from build123d import *

# Parameters (mm, degrees)
F1_DEPTH = 70
F3_DEPTH = 5


with BuildPart() as f1:
    # F0 (on Front) → F1 (new body)
    with BuildSketch(Plane.XZ):
        Polygon((0, 3), (0, 0), (25, 0), (25, -20.415811), (25, -22.415811), (30, -22), (30, 3), align=None)
        Polygon((25, -22.415811), (25, -20.415811), (0, -22.494866), (0, -24.494866), align=None)
    extrude(amount=F1_DEPTH)

    # F2 (on face) → F3 (cut)
    with BuildSketch(Plane.XY.offset(3)):
        with BuildLine():
            ThreePointArc((19, -14.5), (17.828427, -11.671573), (15, -10.5))
            Line((15, -10.5), (15, -14.5))
            Line((15, -14.5), (15, -18.5))
            ThreePointArc((15, -18.5), (17.828427, -17.328427), (19, -14.5))
        make_face()
        with BuildLine():
            ThreePointArc((19, -55.5), (17.828427, -52.671573), (15, -51.5))
            ThreePointArc((15, -51.5), (12.171573, -58.328427), (19, -55.5))
        make_face()
        with BuildLine():
            Line((15, -14.5), (15, -10.5))
            ThreePointArc((15, -10.5), (11, -14.5), (15, -18.5))
            Line((15, -18.5), (15, -14.5))
        make_face()
    extrude(amount=-F3_DEPTH, mode=Mode.SUBTRACT)


solid = f1.part
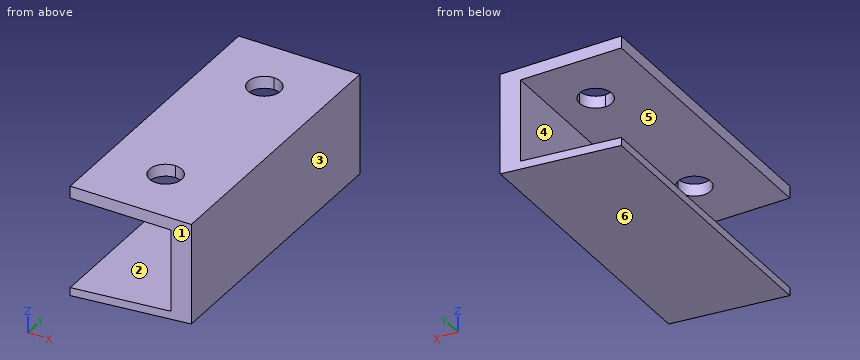
CAD build for the part. Positions are in the model's coordinates, mm. Face numbers are marked on the shaded views. A direction names the side the tool comes from. Give positions to 0.01 mm unless a question says otherwise; leave off trailing zeros. Write each loop counter-clockwise with the first axis right and the second up, starting at its lowest first coordinate (ties: lowest second). Pieces come first, ordered by that corner, then holes. Notation, with made-up numbers: (-19, -26.75) - (0, -26.75) arc R10 ccw to (0, -14.75) - close; hole circle Ø4 at (-18, -25). An arc over 180 degrees is marked (long way). Put each result on its own line as item: value.
(1) Tool access for the marked faces 1 and 2: list every direction of +Z, -Z, +X, -X, +Y, -Y with a clear straight run to the whole face (end or side of a thin tool).
Working result:
face 1: +Z, -Z, +X, -X, -Y
face 2: -X, +Y, -Y
(2) Pull direction Z, two halves, no side cores. Call the marked faces 3, 4, 5 and 6: released by +Z, released by -Z, zero draft, split by the parting line, or undercut.
Working result:
face 3: zero draft
face 4: undercut
face 5: undercut
face 6: released by -Z
(3) Saw through at A-A (x = 6.5). List the corners of the cut face in (y, z), then the cut area to 3 significant figures.
Working result:
outline: (-70, -23.95) - (0, -23.95) - (0, -21.95) - (-70, -21.95) - close; (-70, 0) - (0, 0) - (0, 3) - (-70, 3) - close
area: 350 mm^2
(4) Saw through at D-D (x = 12). List the corners of the cut face in (y, z), then the cut area to 3 significant figures.
Working result:
outline: (-70, -23.5) - (0, -23.5) - (0, -21.5) - (-70, -21.5) - close; (-70, 0) - (-58.15, 0) - (-58.15, 3) - (-70, 3) - close; (-52.85, 0) - (-17.15, 0) - (-17.15, 3) - (-52.85, 3) - close; (-11.85, 0) - (0, 0) - (0, 3) - (-11.85, 3) - close
area: 318 mm^2
(5) Drop flat-ended pins along their axis: pin 1 Ø3 at (x, y) = (17, -17.5) entering from -Z; pin 2 Ø7.5 at (x, y) = (18.5, -26.5) entering from -Z; pin 3 Ø6.5 at (x, y) = (15, -55.5) entering from +Z. Give the stop position or say it passes through.
Working result:
pin 1: z = -23.21
pin 2: z = -23.27
pin 3: z = -20.98
(6) Wall check: L1, parallel to Y at x = 15, z = 2.1; L2, parallel to X at y = -55.5, z = 0.6; L3, parallel to X at y = -33, z = -10. Give the ranges that are in metal, low to high.
Working result:
L1: -70 to -59.5, -51.5 to -18.5, -10.5 to 0
L2: 0 to 11, 19 to 30
L3: 25 to 30
(7) Saw through at C-C (y = -52.5). List the corners of the cut face in (x, z).
Working result:
outline: (0, -24.49) - (30, -22) - (30, 3) - (17.65, 3) - (17.65, 0) - (25, 0) - (25, -20.42) - (0, -22.49) - close; (0, 0) - (12.35, 0) - (12.35, 3) - (0, 3) - close
(8) Saw through at B-B (y = -63). List the corners of the cut face in (x, z), then the cut area to 3 significant figures.
Working result:
outline: (0, -24.49) - (30, -22) - (30, 3) - (0, 3) - (0, 0) - (25, 0) - (25, -20.42) - (0, -22.49) - close
area: 251 mm^2
